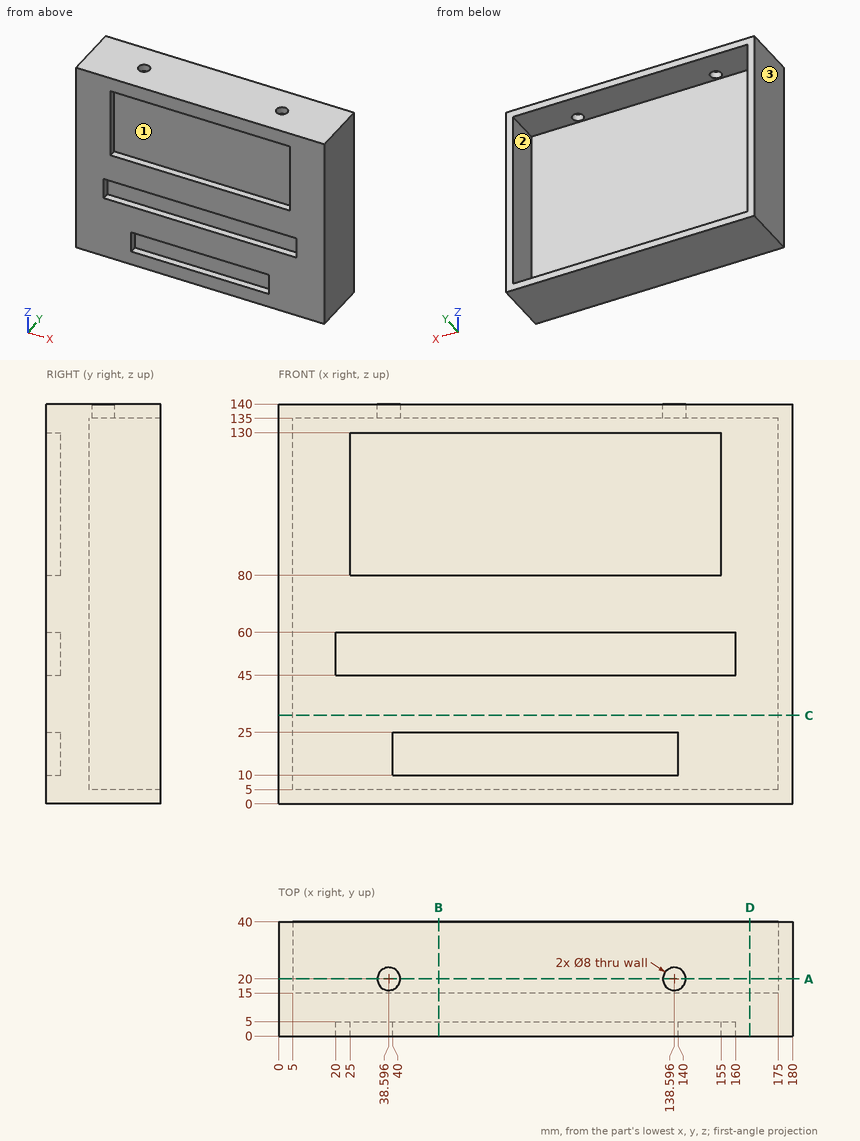
Input: dimensioned drawing with shaded views. Units: mm. Origin: part minimum x, y, z. A direction names the side the tool comes from. Give positions to 0.01 mm unless a question says otherwise; leave off trailing zeros. Loops run counter-clockwise (first coordinate to the right, second up) from the corner with the lowest first, then second, coordinate; pieces in that order, holes last. Notation, with made-up numbers: M 7,-19 L 34,-19 A25 ccw 34,-7 Z; hole C 33,36 d9. An arc over 180 degrees is marked long. Put each result on its own line as item: value. Start each with the question number.
1) Contact query for flat-ended pins moving along their axis: pin 1 (4 mm diameter, centred on y = 2.5, z = 55.5, fed in from -X); pin 2 (15 mm diameter, centred on x = 92.5, z = 106, fed in from -Y). Output: stop coordinate, or through.
2) Cut plane B-B (x = 56). Output: boundary loops of the cut face in (y, z), then the cut area to 3 significant figures.
3) Ray query, line 1 along Z through (x, y) = (33, 38); line 2 along X through (y, z) = (4, 58); line 3 along X through (y, z) = (37.5, 117). Return the intervals inside material, ascending.
4) Cut plane D-D (x = 165). Output: boundary loops of the cut face in (y, z).
5) Cut plane C-C (z = 31). Output: boundary loops of the cut face in (x, y).
6) Access query for the marked faces 1, 2 and 3. Directions: +Z, -Z, +X, -X, +Y, -Y. A direction counts if a zero-diameter tool reaches every point of the face in a straight line with its end or side. Return the directions, or none.
7) Cut plane A-A (y = 20). Output: boundary loops of the cut face in (x, z), then the cut area to 3 significant figures.
Verdict:
1. pin 1: x = 0
1. pin 2: y = 5
2. outline: M 0,0 L 40,0 L 40,5 L 15,5 L 15,135 L 40,135 L 40,140 L 0,140 L 0,130 L 5,130 L 5,80 L 0,80 L 0,60 L 5,60 L 5,45 L 0,45 L 0,25 L 5,25 L 5,10 L 0,10 Z
2. area: 1,950 mm2
3. line 1: 0 to 5, 135 to 140
3. line 2: 0 to 20, 160 to 180
3. line 3: 0 to 5, 175 to 180
4. outline: M 0,0 L 40,0 L 40,5 L 15,5 L 15,135 L 40,135 L 40,140 L 0,140 Z
5. outline: M 0,0 L 180,0 L 180,40 L 175,40 L 175,15 L 5,15 L 5,40 L 0,40 Z
6. face 1: -Y
6. face 2: +Y
6. face 3: +Z, -Z, -X, +Y, -Y
7. outline: M 0,0 L 180,0 L 180,140 L 142.6,140 L 142.6,135 L 175,135 L 175,5 L 5,5 L 5,135 L 34.6,135 L 34.6,140 L 0,140 Z; M 42.6,135 L 134.6,135 L 134.6,140 L 42.6,140 Z
7. area: 3,020 mm2
